Build history of the part. All positions in model axes, mm. Face numbers are marked on the shaded views. A direction names the side the tool comes from. Coordinates: 2 decimals unless noted, no trailing zeros. Loops run counter-clockwise (first coordinate to the right, second up) from the corner with the lowest first, then second, coordinate; pieces in that order, holes last.
Item 1: Flat gauge pin, fed straight in: pin 1 (4 mm diameter, centred on x = 47.5, z = 20, fed in from -Y). Where does the tip first touch, or does it go through?
Item 2: Cut at C-C (x = -47). List the corners of the cut face in (y, z).
Item 3: Cut at B-B (y = 68). List the corners of the cut face in (x, z).
Item 4: Drill centre lines: line 1 along Y through (x, z) = (-90, 11); line 2 along Y through (x, z) = (-38.5, 22.75). Where is each one in solid material? Low to high.
Item 5: Cut at A-A (z = 14.25). List the corners of the cut face in (x, y).
Item 6: 3-axis set-ups, long thin cutter, end or side, ignore diameter. For the marked faces 1 and 2: which of +Z, -Z, +X, -X, +Y, -Y reach the whole face in a straight line?
from build123d import *

# Parameters (mm, degrees)
SKETCH1_W           = 254
SKETCH1_H           = 177.8
BOSS_EXTRUDE1_DEPTH = 25.4
CUT_EXTRUDE1_DEPTH  = 158.090324336


with BuildPart() as part:
    # Sketch1 → Boss-Extrude1 (new body)
    with BuildSketch(Plane.XY):
        Rectangle(SKETCH1_W, SKETCH1_H)
    extrude(amount=BOSS_EXTRUDE1_DEPTH)

    # Sketch3 → Cut-Extrude1 (cut, through all)
    with BuildSketch(Plane.XY.offset(25.4)):
        Polygon((127, 88.9), (-49.53, 88.9), (127, 37.598007728), align=None)
        Polygon((-49.53, 83.82), (-127, 83.82), (-127, -88.9), (127, -88.9), (127, 37.598007728), (109.519735389, 37.598007728), align=None)
    extrude(amount=-CUT_EXTRUDE1_DEPTH, mode=Mode.SUBTRACT)


solid = part.part
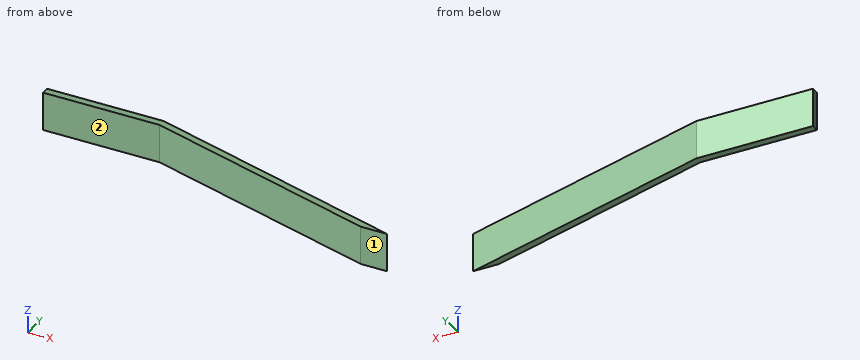
Filled sheet:
1. pin 1: stops at y = 55.04
2. outline: (83.08, 0) - (88.16, 0) - (88.16, 25.4) - (83.08, 25.4) - close
3. outline: (4.91, 0) - (22.39, 0) - (22.39, 25.4) - (4.91, 25.4) - close
4. line 1: y = 83.82 to 88.9
4. line 2: y = 80.61 to 85.69
5. outline: (-127, 83.82) - (-49.53, 83.82) - (109.52, 37.6) - (127, 37.6) - (-49.53, 88.9) - (-127, 88.9) - close
6. face 1: +Z, -Z, +X, -X, -Y
6. face 2: +Z, -Z, -X, -Y
